Check sheet for the drawn part. Datum: minimum x, y, z corner. Units: mm. A direction names the side the tool comes from. Coordinates: 2 decimals unless noted, no trailing zeros. Write each loop counter-clockwise with the first axis right and the second up, starting at its lowest first coordinate (ties: lowest second). Pieces come first, ordered by that corner, then holes. Notation, with made-up numbers: (-40, 28.25) - (-15, 28.25) arc R18 cw to (-15, 51.25) - close; hole circle Ø8 at (83.5, 81.25). An arc over 180 degrees is marked (long way). Write each question's results on one line, items separated by ' | '.
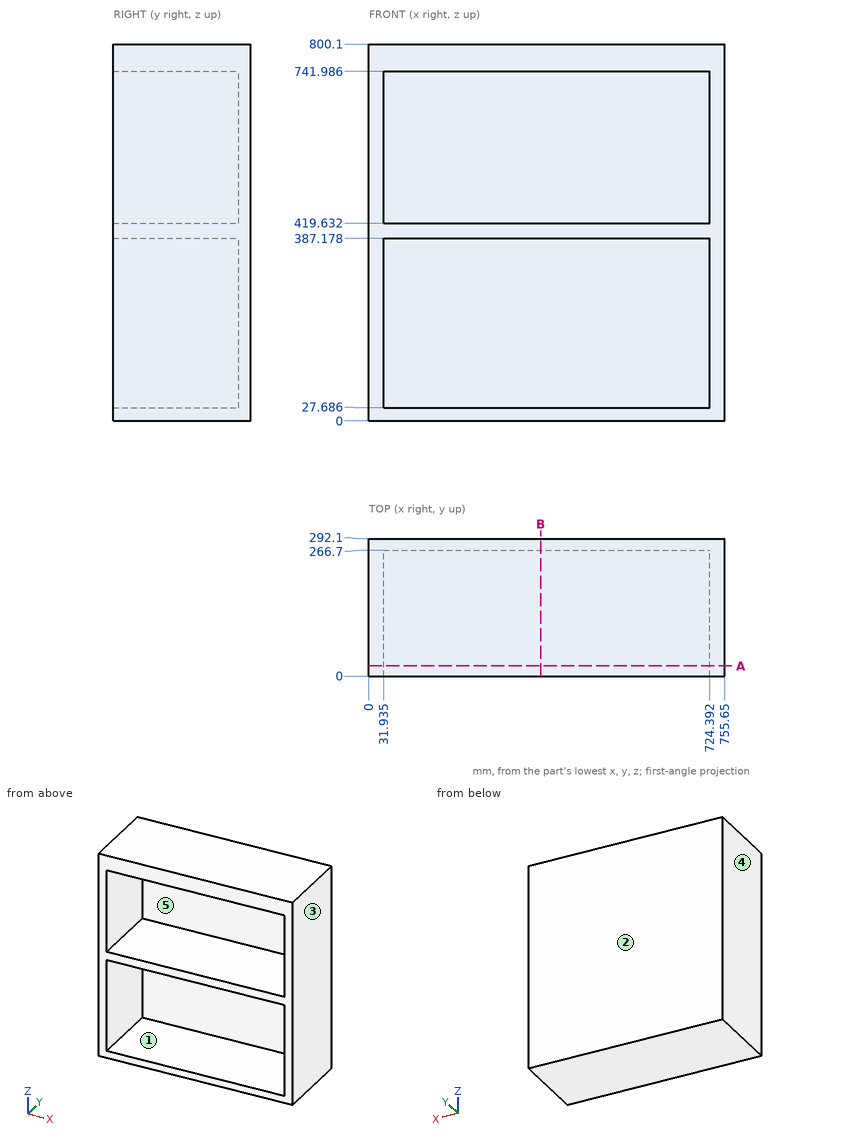
1. Access from +Z, -Z, +X, -X, +Y, -Y to the whole of each face (thin tool, end or side, straight path). Record for the marked faces 1 and 2.
Values follow:
face 1: -Y | face 2: +Z, -Z, +X, -X, +Y
2. Material ranges on L1, parallel to Z at x = 212, y = 47 (1 decimal); L2, parallel to Y at x = 709, z = 271, recorded low to high. Write a range as [from, to].
Values follow:
L1: z = [0, 27.7], [387.2, 419.6], [742, 800.1] | L2: y = [266.7, 292.1]
3. Draft check along X on the marked faces 3, 4 and 5. Enter one of: pulls with the +X half, pulls with the -X half, needs draft (parallel to the pull), parting line crosses it, or undercut.
Values follow:
face 3: pulls with the +X half | face 4: pulls with the -X half | face 5: undercut
4. Sectioned sample at A-A (y = 21.5). Give the number of separate pieces and of enclosed holes in the cut face, then the cut area to 3 significant figures.
Values follow:
separate pieces: 1 | enclosed holes: 2 | area: 132,000 mm^2
5. Go/stop test with a flat-tipped pin: pin 1 (10 mm diameter, centred on x = 99, z = 444, fed in from -Y). Record where the tip stops, or that it passes through.
Values follow:
pin 1: stops at y = 266.7
6. Sectioned sample at B-B (x = 365). Record the cut outline in (y, z) (1 decimal), then the cut area to 3 significant figures.
Values follow:
outline: (0, 0) - (292.1, 0) - (292.1, 800.1) - (0, 800.1) - (0, 742) - (266.7, 742) - (266.7, 419.6) - (0, 419.6) - (0, 387.2) - (266.7, 387.2) - (266.7, 27.7) - (0, 27.7) - close | area: 51,900 mm^2
